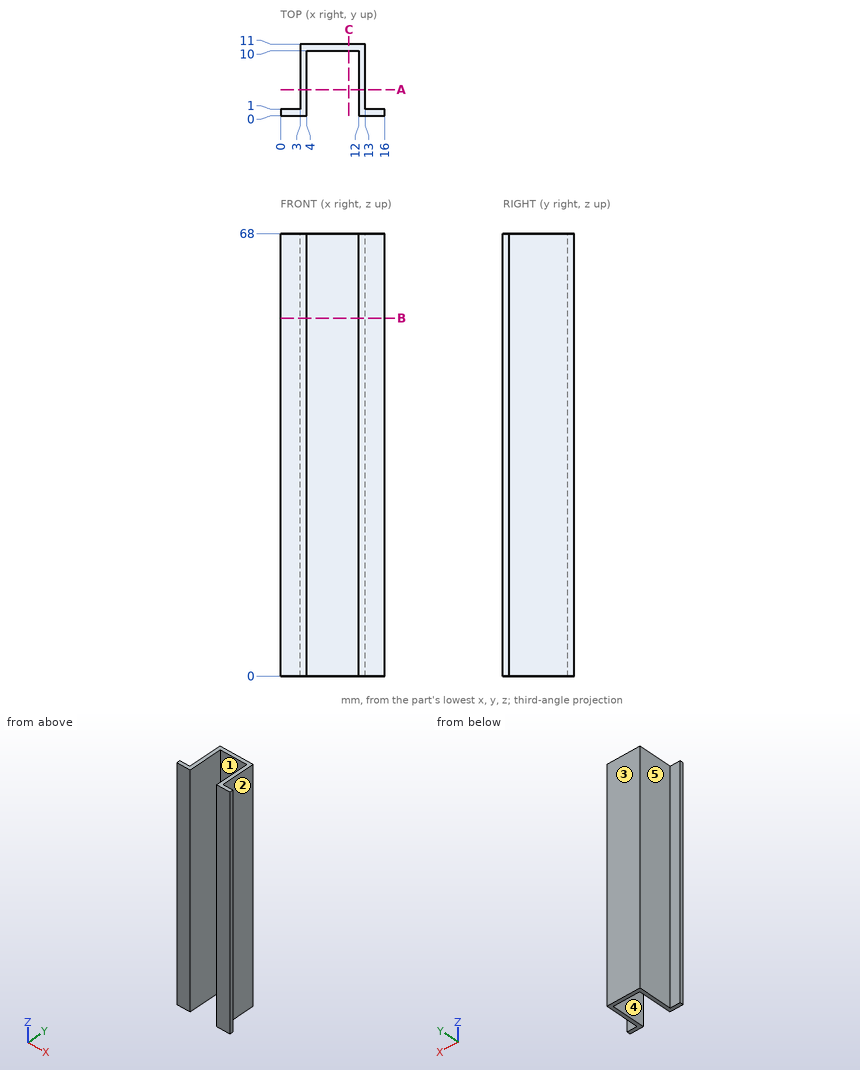
The drawing under review shows one solid part. Ordinate dimensions are in mm from its lowest x, y, z. A direction names the side the tool comes from. Round coordinates to 2 decimals unless told otherwise and drop trailing zeros. Loops run counter-clockwise (first coordinate to the right, second up) from the corner with the lowest first, then second, coordinate; pieces in that order, holes last. Notation, with made-up numbers: (-8.5, 55.25) - (37.5, 55.25) arc R11 ccw to (37.5, 76.25) - close; hole circle Ø10 at (57, 11.25). An arc over 180 degrees is marked (long way). Use one line per item in the form item = value.
Item 1: Clearance check with flat-ended pins moving along their axes: P1, Ø9, axis at x = 6.5, z = 50, coming from the -Y side; P2, Ø5, axis at y = 8, z = 25.5, coming from the +X side; P3, Ø4, axis at y = 6, z = 12, coming from the -X side; P4, Ø1.5, axis at x = 14, z = 17.5, coming from the +Y side. State where each tip first meets the part, or that it passes through.
Answers:
P1 = 0
P2 = 13
P3 = 3
P4 = 1
Item 2: Tool access review of the marked faces 1 and 2: name each direction out of +Z, -Z, +X, -X, +Y, -Y from which nothing blocks a thin tool from reaching the whole face with its end or side.
Answers:
face_1 = +Z, -Z, -Y
face_2 = +Z, -Z, +X, +Y
Item 3: For line 1 (X direction, y = 4.5, z = 61); line 2 (Y direction, x = 7.75, z = 10); line 3 (Y direction, x = 1.25, z = 22), list the stretches that pass through material, from the lowest coordinate up.
Answers:
line_1 = 3 to 4, 12 to 13
line_2 = 10 to 11
line_3 = 0 to 1
Item 4: Consider section A-A on y = 4. Write out the cut boundary in (x, z).
Answers:
outline = (3, 0) - (4, 0) - (4, 68) - (3, 68) - close; (12, 0) - (13, 0) - (13, 68) - (12, 68) - close
Item 5: Consider section B-B on z = 55. Write out the cut boundary in (x, y).
Answers:
outline = (0, 0) - (4, 0) - (4, 10) - (12, 10) - (12, 0) - (16, 0) - (16, 1) - (13, 1) - (13, 11) - (3, 11) - (3, 1) - (0, 1) - close
Item 6: Consider section C-C on x = 10.5. Write out the cut boundary in (y, z), then the cut area to 3 significant figures.
Answers:
outline = (10, 0) - (11, 0) - (11, 68) - (10, 68) - close
area = 68.0 mm^2
Item 7: Mouldability with a two-part tool opening along X and no side actions: class the marked faces 3, 4 and 5 as +X half, -X half, draft (parallel to the pull), parting line (faces both ways), or undercut.
Answers:
face_3 = draft
face_4 = undercut
face_5 = -X half
